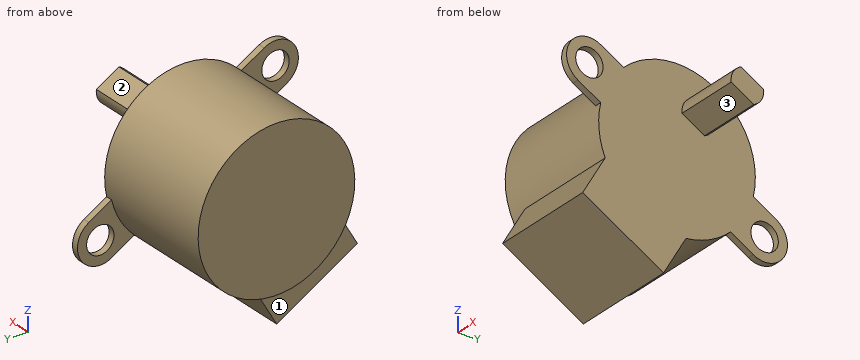
from build123d import *

# Parameters (mm, degrees)
SKETCH034_R             = 12
PAD014_DEPTH            = 19
SKETCH035_W             = 14.3
SKETCH035_H             = 10
PAD015_DEPTH            = 16.3
SKETCH036_R             = 2.1
PAD016_DEPTH            = 1
PAD017_DEPTH            = 10
BODY007_ROLL_ANGLE      = 90
BODY007_PITCH_ANGLE     = 30
BODY007_PLACEMENT_ANGLE = 90


with BuildPart() as part:
    # Sketch034 → Pad014 (new body)
    with BuildSketch(Plane.XY):
        Circle(SKETCH034_R)
    extrude(amount=PAD014_DEPTH)

    # Sketch035 (on Face3 of Pad014) → Pad015 (join)
    with BuildSketch(Plane.XY.offset(19)):
        with Locations((0, -11.5)):
            Rectangle(SKETCH035_W, SKETCH035_H)
    extrude(amount=-PAD015_DEPTH)

    # Sketch036 (on Face3 of Pad015) → Pad016 (join)
    with BuildSketch(Plane.XY.offset(19)):
        with BuildLine():
            ThreePointArc((15.5, -3.5), (19, 0), (15.5, 3.5))
            Line((15.5, 3.5), (-15.5, 3.5))
            ThreePointArc((-15.5, 3.5), (-19, 0), (-15.5, -3.5))
            Line((-15.5, -3.5), (15.5, -3.5))
        make_face()
        with Locations((15.5, 0)):
            Circle(SKETCH036_R, mode=Mode.SUBTRACT)
        with Locations((-15.5, 0)):
            Circle(SKETCH036_R, mode=Mode.SUBTRACT)
    extrude(amount=-PAD016_DEPTH)

    # Sketch037 (on Face11 of Pad016) → Pad017 (join)
    with BuildSketch(Plane.XY.offset(19)):
        with BuildLine():
            ThreePointArc((-2, 8), (-2.5, 6.5), (-2, 5))
            Line((-2, 5), (2, 5))
            ThreePointArc((2, 5), (2.5, 6.5), (2, 8))
            Line((-2, 8), (2, 8))
        make_face()
    extrude(amount=PAD017_DEPTH)


with BuildPart() as part_1:
    # Body007 roll: moved
    add(part.part.rotate(Axis((0, 0, 0), (1, 0, 0)), BODY007_ROLL_ANGLE))


with BuildPart() as part_2:
    # Body007 pitch: moved
    add(part_1.part.rotate(Axis((0, 0, 0), (0, 1, 0)), BODY007_PITCH_ANGLE))


with BuildPart() as part_3:
    # Body007 placement: moved
    add(part_2.part.moved(Location((20.005183, -14.807107, -27.2))).rotate(Axis((20.005183, -14.807107, -27.2), (0, 0, 1)), BODY007_PLACEMENT_ANGLE))


solid = part_3.part
The model under review builds one solid part; all positions refer to its coordinate system, in mm. Face numbers are marked on the shaded views. A direction names the side the tool comes from. Round coordinates to 2 decimals unless told otherwise and drop trailing zeros. Loops run counter-clockwise (first coordinate to the right, second up) from the corner with the lowest first, then second, coordinate; pieces in that order, holes last. Notation, with made-up numbers: M -29,63.5 L 9,63.5 A19 cw 9,70.5 Z; hole C 23,-27.75 d11. An arc over 180 degrees is marked long. Answer as CSV lines item,"result". Start each with the question number.
Item 1: For the marked faces 1, 2 and 3, list the 3-axis set-ups (+Z, -Z, +X, -X, +Y, -Y) from which the entire face can be reached by the end or side of a thin tool; tool diameter is ignored.
Item 2: Insertion check: P1, Ø6.5, axis at y = -28.23, z = -19.45, coming from the -X side; P2, Ø1, axis at x = 23, y = -20.5, coming from the +Z side; P3, Ø1, axis at x = 30, z = -36.5, coming from the -Y side. Each pin has a flat end and moves straight along its axis. Give the tip position at first contact, or say it passes through.
Item 3: Consider section D-D (z = -30.75). Write out the cut boundary in (x, y), then the cut area to 3 significant figures.
Item 4: Consider section C-C (x = 41.5). Write out the cut boundary in (y, z), then the cut area to 3 significant figures.
Item 5: Consider section B-B (y = -13). Write out the cut boundary in (x, z), then the cut area to 3 significant figures.
Item 6: Wall thickness on line 1 (X direction, y = -17, z = -17.75); line 2 (X direction, y = -18.5, z = -39.25); line 3 (Y direction, x = 38.5, z = -19.45): over which ranges is each line inside the solid? List them lowest first. Write a range as [from, to].
Item 7: Consider section A-A (z = -34.95). Write out the cut boundary in (x, y), then the cut area to 3 significant figures.
Answer:
1,face 1,"-Z, -X, -Y"
1,face 2,"+Z, +X, +Y"
1,face 3,"-Z, +X, -Y"
2,P1,"stops at x = 38.01"
2,P2,"stops at z = -16.38"
2,P3,"stops at y = -28.72"
3,outline,"M 20.01,-26.27 L 39.01,-26.27 L 39.01,-1.66 L 38.01,-1.66 L 38.01,-3.34 L 20.01,-3.34 Z"
3,area,"437 mm^2"
4,outline,"M -14.04,-21.87 L -10.58,-23.87 A2.5 ccw -9.08,-21.27 L -12.54,-19.27 A2.5 ccw Z"
4,area,"14.0 mm^2"
5,outline,"M 20.01,-39.06 L 39.01,-39.06 L 39.01,-22.47 L 49.01,-22.47 L 49.01,-19.53 L 39.01,-19.53 L 39.01,-15.34 L 20.01,-15.34 Z"
5,area,"480 mm^2"
6,line 1,"x = [20.01, 39.01]"
6,line 2,"x = [22.71, 39.01]"
6,line 3,"y = [-31.73, -30.33], [-26.13, -5.65]"
7,outline,"M 20.01,-23.97 L 22.71,-23.97 L 22.71,-27.54 L 39.01,-27.54 L 39.01,-3.48 L 38.01,-3.48 L 38.01,-5.65 L 20.01,-5.65 Z; M 38.01,0.72 L 39.01,0.72 L 39.01,2.12 L 38.01,2.12 Z"
7,area,"410 mm^2"
